Source: CAD feature listing. Evaluate the final solid. Frame: model axes, mm. Coordinates: 2 decimals unless noted, no trailing zeros. Order: outer loops, then holes, each group sorted by start corner. A loop starts at its lowest first (then second) coordinate and runs counter-clockwise, first axis right, second up. Notation, with made-up numbers: (67.25, -35.5) -> (91.25, -35.5) arc R16 ccw to (91.25, -12.5) -> close; hole circle Ø9 at (18, -4.5). An arc over 180 degrees is marked (long way). Write item = value, one per line. Start each with the question number.
Item 1: Ray query, line 1 along X through (y, z) = (1.4, -5); line 2 along X through (y, z) = (1.45, -6.25); line 3 along Z through (x, y) = (32, 1.7). Return the intervals inside material, ascending. Write a range as [from, to].
Item 2: Section query C-C (x = 30). Output: boundary loops of the cut face in (y, z).
Item 3: Section query A-A (z = -5). Output: boundary loops of the cut face in (x, y), then the cut area to 3 significant figures.
Item 4: Section query B-B (x = 4). Output: boundary loops of the cut face in (y, z).
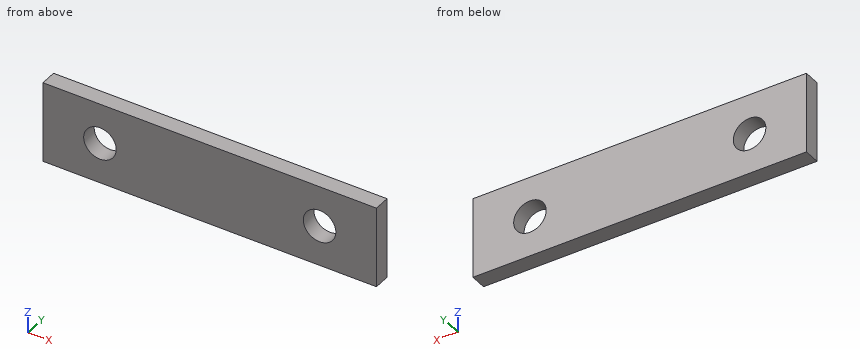
```python
from build123d import *

# Parameters (mm, degrees)
SKETCH1_W           = 35
SKETCH1_H           = 10
BOSS_EXTRUDE1_DEPTH = 2
SKETCH4_R           = 2
CUT_EXTRUDE2_DEPTH  = 20
SKETCH5_W           = 10
SKETCH5_H           = 2
BOSS_EXTRUDE3_DEPTH = 3
SKETCH6_W           = 10
SKETCH6_H           = 2
BOSS_EXTRUDE4_DEPTH = 3


with BuildPart() as part:
    # Sketch1 → Boss-Extrude1 (new body)
    with BuildSketch(Plane(origin=(0, 0, 0), x_dir=(1, 0, 0), z_dir=(0, 1, 0))):
        with Locations((17.5, 5)):
            Rectangle(SKETCH1_W, SKETCH1_H)
    extrude(amount=BOSS_EXTRUDE1_DEPTH)

    # Sketch4 → Cut-Extrude2 (cut)
    with BuildSketch(Plane.XZ):
        with Locations(Location((4, -5, 0), (0, 0, 270))):
            Circle(SKETCH4_R)
        with Locations(Location((31, -5, 0), (0, 0, 270))):
            Circle(SKETCH4_R)
    extrude(amount=-CUT_EXTRUDE2_DEPTH, mode=Mode.SUBTRACT)

    # Sketch5 → Boss-Extrude3 (add)
    with BuildSketch(Plane.ZY):
        with Locations((-5, 1)):
            Rectangle(SKETCH5_W, SKETCH5_H)
    extrude(amount=BOSS_EXTRUDE3_DEPTH)

    # Sketch6 → Boss-Extrude4 (add)
    with BuildSketch(Plane(origin=(35, 0, 0), x_dir=(0, 0, -1), z_dir=(1, 0, 0))):
        with Locations((5, 1)):
            Rectangle(SKETCH6_W, SKETCH6_H)
    extrude(amount=BOSS_EXTRUDE4_DEPTH)


solid = part.part
```
Computed:
q1.line_1 = [-3, 2], [6, 29], [33, 38]
q1.line_2 = [-3, 2.44], [5.56, 29.44], [32.56, 38]
q1.line_3 = [-10, -6.73], [-3.27, 0]
q2.outline = (0, -10) -> (2, -10) -> (2, -6.73) -> (0, -6.73) -> close; (0, -3.27) -> (2, -3.27) -> (2, 0) -> (0, 0) -> close
q3.outline = (-3, 0) -> (2, 0) -> (2, 2) -> (-3, 2) -> close; (6, 0) -> (29, 0) -> (29, 2) -> (6, 2) -> close; (33, 0) -> (38, 0) -> (38, 2) -> (33, 2) -> close
q3.area = 66.0 mm^2
q4.outline = (0, -10) -> (2, -10) -> (2, -7) -> (0, -7) -> close; (0, -3) -> (2, -3) -> (2, 0) -> (0, 0) -> close
